```python
from build123d import *

# Parameters (mm, degrees)
F1_DEPTH    = 6.35
F2_SIZE2    = 0.1791482124
F2_SIZE     = 1.016
F2_2_SIZE2  = 0.1791482124
F2_2_SIZE   = 1.016
F2_3_SIZE2  = 0.1791482124
F2_3_SIZE   = 1.016
F3_SIZE2    = 0.1791482124
F3_SIZE     = 1.016
F4_SIZE2    = 0.6805909488
F4_SIZE     = 2.54
F5_SIZE2    = 0.6805909488
F5_SIZE     = 2.54
F6_T4_DEPTH = 18.0529676813


# Not quite as in the source:
# - a fillet or chamfer that OpenCascade refuses, or shapes differently, is made with other operations: its cross-section is extruded or revolved along the edge and cut away or added


with BuildPart() as f1:
    # F0 (on Right) → F1 (new body)
    with BuildSketch(Plane.YZ):
        with BuildLine():
            Line((0, 1.27), (0, 0))
            Line((0, 0), (38.1, 0))
            Line((38.1, 0), (38.1, 1.27))
            ThreePointArc((38.1, 1.27), (37.7280256121, 2.1680256121), (36.83, 2.54))
            Line((36.83, 2.54), (28.575, 2.54))
            Line((28.575, 2.54), (28.575, 3.81))
            Line((28.575, 3.81), (23.495, 3.81))
            Line((23.495, 3.81), (23.495, 2.54))
            Line((23.495, 2.54), (18.415, 2.54))
            Line((18.415, 2.54), (18.415, 3.81))
            Line((18.415, 3.81), (16.51, 3.81))
            Line((16.51, 3.81), (16.51, 2.54))
            Line((16.51, 2.54), (11.43, 2.54))
            Line((11.43, 2.54), (11.43, 3.81))
            Line((11.43, 3.81), (9.525, 3.81))
            Line((9.525, 3.81), (9.525, 2.54))
            Line((9.525, 2.54), (1.27, 2.54))
            ThreePointArc((1.27, 2.54), (0.3719743879, 2.1680256121), (0, 1.27))
        make_face()
    extrude(amount=F1_DEPTH)

    # F2
    f2_edges = [f1.edges().sort_by_distance(p)[0] for p in [
        (3.175, 11.43, 3.81),
    ]]
    f2_side = f1.faces().sort_by_distance((3.175, 11.43, 3.175))[0]
    chamfer(f2_edges, length=F2_SIZE, length2=F2_SIZE2, reference=f2_side)

    # F2#2
    f2_2_edges = [f1.edges().sort_by_distance(p)[0] for p in [
        (3.175, 9.525, 3.81),
    ]]
    f2_2_side = f1.faces().sort_by_distance((3.175, 9.525, 3.175))[0]
    chamfer(f2_2_edges, length=F2_2_SIZE, length2=F2_2_SIZE2, reference=f2_2_side)

    # F2#3
    f2_3_edges = [f1.edges().sort_by_distance(p)[0] for p in [
        (3.175, 18.415, 3.81),
    ]]
    f2_3_side = f1.faces().sort_by_distance((3.175, 18.415, 3.175))[0]
    chamfer(f2_3_edges, length=F2_3_SIZE, length2=F2_3_SIZE2, reference=f2_3_side)

    # F3
    f3_edges = [f1.edges().sort_by_distance(p)[0] for p in [
        (3.175, 16.51, 3.81),
    ]]
    f3_side = f1.faces().sort_by_distance((3.175, 16.51, 3.175))[0]
    chamfer(f3_edges, length=F3_SIZE, length2=F3_SIZE2, reference=f3_side)

    # F4
    f4_edges = [f1.edges().sort_by_distance(p)[0] for p in [
        (6.35, 10.4775, 3.81),
    ]]
    f4_side = f1.faces().sort_by_distance((6.35, 19.258705, 1.457125))[0]
    chamfer(f4_edges, length=F4_SIZE, length2=F4_SIZE2, reference=f4_side)

    # F5
    f5_edges = [f1.edges().sort_by_distance(p)[0] for p in [
        (0, 17.4625, 3.81),
    ]]
    f5_side = f1.faces().sort_by_distance((0, 19.258705, 1.457125))[0]
    chamfer(f5_edges, length=F5_SIZE, length2=F5_SIZE2, reference=f5_side)

    # F6: chamfer of 2.54 on 1 edges, made by hand


with BuildPart() as f6_tool2:
    # F6_s3 → F6_t4 (new body)
    with BuildSketch(Plane.YZ.offset(-5.8514838407)):
        Polygon((28.575, 1.27), (26.035, 3.81), (28.575, 3.81), align=None)
    extrude(amount=F6_T4_DEPTH)

    split(bisect_by=Plane.XY.offset(2.54), keep=Keep.TOP)


with BuildPart() as f1_1:
    add(f1.part)

    # F6_t1: cut F6_tool2
    add(f6_tool2.part, mode=Mode.SUBTRACT)


solid = f1_1.part
```
The model under review builds one solid part; all positions refer to its coordinate system, in mm. A direction names the side the tool comes from. Round coordinates to 2 decimals unless told otherwise and drop trailing zeros. Order: outer loops, then holes, each group sorted by start corner. A loop starts at its lowest first (then second) coordinate and runs counter-clockwise, first axis right, second up. Notation, with made-up numbers: (4, 50.5) -> (51, 50.5) arc R22 cw to (51, 65.5) -> close; hole circle Ø11 at (-33.75, -17). An arc over 180 degrees is marked (long way). Use a Markdown table: item, result.
Q1. Clearance check with flat-ended pins moving along their axes: P1, Ø1, axis at x = 4.5, z = 2.5, coming from the +Y side; P2, Ø3, axis at x = 5.5, y = 34, coming from the +Z side; P3, Ø0.6, axis at x = 4, z = 3, coming from the -Y side (3 decimals). State where each tip first meets the part, or that it passes through.
Values:
| item | result |
|---|---|
| P1 | stops at y = 37.87 |
| P2 | stops at z = 2.54 |
| P3 | stops at y = 9.525 |
Q2. We need section A-A on x = 5. Write out the cut boundary in (y, z) (3 decimals), then the cut area to 3 significant figures.
Values:
| item | result |
|---|---|
| outline | (0, 0) -> (38.1, 0) -> (38.1, 1.27) arc R1.27 ccw to (36.83, 2.54) -> (27.305, 2.54) -> (26.035, 3.81) -> (23.495, 3.81) -> (23.495, 2.54) -> (18.415, 2.54) -> (18.415, 2.794) -> (18.236, 3.81) -> (16.689, 3.81) -> (16.51, 2.794) -> (16.51, 2.54) -> (11.43, 2.54) -> (11.43, 2.794) -> (11.251, 3.81) -> (9.704, 3.81) -> (9.525, 2.794) -> (9.525, 2.54) -> (1.27, 2.54) arc R1.27 ccw to (0, 1.27) -> close |
| area | 105 mm^2 |
Q3. Tool access review of faces 1 (the flat face through (3, 5, 2.54)), 2 (the flat face through (3, 32, 2.54)), 3 (the flat face through (3.1, 16.6, 3.3)), 4 (the flat face through (3, 38.1, 1)), 5 (the flat face through (6.35, 19, 1)): name each direction out of +Z, -Z, +X, -X, +Y, -Y from which nothing blocks a thin tool from reaching the whole face with its end or side.
Values:
| item | result |
|---|---|
| face 1 | +Z, +X, -X, -Y |
| face 2 | +Z, +X, -X, +Y |
| face 3 | +Z, +X, -X |
| face 4 | +Z, -Z, +X, -X, +Y |
| face 5 | +Z, -Z, +X, +Y, -Y |
Q4. For line 1 (Z direction, x = 3, y = 31); line 2 (Y direction, x = 1.5, z = 3) (3 decimals); line 3 (Y direction, x = 4.25, z = 1.35), list the stretches that pass through material, from the lowest coordinate up.
Values:
| item | result |
|---|---|
| line 1 | z = 0 to 2.54 |
| line 2 | y = 9.561 to 11.394, 16.546 to 18.379, 23.495 to 26.845 |
| line 3 | y = 0 to 38.1 |
Q5. We need section D-D on y = 20.5. Write out the cut boundary in (x, z).
Values:
| item | result |
|---|---|
| outline | (0, 0) -> (6.35, 0) -> (6.35, 1.27) -> (6.01, 2.54) -> (0.34, 2.54) -> (0, 1.27) -> close |
Q6. We need section B-B on y = 25. Write out the cut boundary in (x, z).
Values:
| item | result |
|---|---|
| outline | (0, 0) -> (6.35, 0) -> (6.35, 1.27) -> (5.67, 3.81) -> (0.68, 3.81) -> (0, 1.27) -> close |
Q7. We need section C-C on z = 1.6. Write out the cut boundary in (x, y).
Values:
| item | result |
|---|---|
| outline | (0.09, 0.04) -> (6.26, 0.04) -> (6.26, 38.06) -> (0.09, 38.06) -> close |
Q8. Mouldability with a two-part tool opening along Y and no side actions: class faces 6 (the flat face through (3.136, 18.324, 3.309)), 7 (the flat face through (3.135, 26.679, 3.166)), 8 (the flat face through (0.194, 19.317, 1.993)) as +Y half, -Y half, draft (parallel to the pull), parting line (faces both ways), or undercut.
Values:
| item | result |
|---|---|
| face 6 | undercut |
| face 7 | +Y half |
| face 8 | draft |
